from build123d import *

# Parameters (mm, degrees)
ESQUISSE1_W                = 393.7
ESQUISSE1_H                = 95.25
BOSS_EXTRU_1_DEPTH         = 6.35
ESQUISSE2_W                = 38.1
ESQUISSE2_H                = 6.35
ENL_V_MAT_EXTRU_1_DEPTH    = 6.35
ESQUISSE3_W                = 38.1
ESQUISSE3_H                = 6.35
ENL_V_MAT_EXTRU_2_DEPTH    = 6.35
R_P_TITION_LIN_AIRE1_COUNT = 4
R_P_TITION_LIN_AIRE1_PITCH = 76.2
SYM_TRIE2_COPY_1_SKETCH_W  = 38.1
SYM_TRIE2_COPY_1_SKETCH_H  = 6.35
SYM_TRIE2_COPY_1_DEPTH     = 6.35
SYM_TRIE2_COPY_2_SKETCH_W  = 38.1
SYM_TRIE2_COPY_2_SKETCH_H  = 6.35
SYM_TRIE2_COPY_2_DEPTH     = 6.35
SYM_TRIE2_COPY_3_SKETCH_W  = 38.1
SYM_TRIE2_COPY_3_SKETCH_H  = 6.35
SYM_TRIE2_COPY_3_DEPTH     = 6.35


with BuildPart() as part:
    # Esquisse1 → Boss.-Extru.1 (new body)
    with BuildSketch(Plane(origin=(0, 0, 0), x_dir=(1, 0, 0), z_dir=(0, 1, 0))):
        Rectangle(ESQUISSE1_W, ESQUISSE1_H)
    extrude(amount=BOSS_EXTRU_1_DEPTH)

    # Esquisse2 → Enlèv. mat.-Extru.1 (cut)
    with BuildSketch(Plane.ZY.offset(196.85)):
        with Locations((0, 3.175)):
            Rectangle(ESQUISSE2_W, ESQUISSE2_H)
    enl_v_mat_extru_1 = extrude(amount=-ENL_V_MAT_EXTRU_1_DEPTH, mode=Mode.SUBTRACT)

    # Symétrie1: Enlèv. mat.-Extru.1 across plane
    add(enl_v_mat_extru_1.mirror(Plane(origin=(0, 0, 0), x_dir=(0, 0, 1), z_dir=(1, 0, 0))), mode=Mode.SUBTRACT)

    # Esquisse3 → Enlèv. mat.-Extru.2 (cut)
    with BuildSketch(Plane(origin=(0, 0, -47.625), x_dir=(-1, 0, 0), z_dir=(0, 0, -1))):
        with Locations((114.3, 3.175)):
            Rectangle(ESQUISSE3_W, ESQUISSE3_H)
    enl_v_mat_extru_2 = extrude(amount=-ENL_V_MAT_EXTRU_2_DEPTH, mode=Mode.SUBTRACT)

    # Répétition linéaire1: Enlèv. mat.-Extru.2 ×4
    with Locations(*[(i * R_P_TITION_LIN_AIRE1_PITCH, 0, 0) for i in range(1, R_P_TITION_LIN_AIRE1_COUNT)]):
        add(enl_v_mat_extru_2, mode=Mode.SUBTRACT)

    # Symétrie2: Enlèv. mat.-Extru.2 across plane
    add(enl_v_mat_extru_2.mirror(Plane.XY), mode=Mode.SUBTRACT)

    # Symétrie2 copy 1 sketch → Symétrie2 copy 1 (cut)
    with BuildSketch(Plane(origin=(76.2, 0, 47.625), x_dir=(-1, 0, 0), z_dir=(0, 0, 1))):
        with Locations((114.3, -3.175)):
            Rectangle(SYM_TRIE2_COPY_1_SKETCH_W, SYM_TRIE2_COPY_1_SKETCH_H)
    extrude(amount=-SYM_TRIE2_COPY_1_DEPTH, mode=Mode.SUBTRACT)

    # Symétrie2 copy 2 sketch → Symétrie2 copy 2 (cut)
    with BuildSketch(Plane(origin=(152.4, 0, 47.625), x_dir=(-1, 0, 0), z_dir=(0, 0, 1))):
        with Locations((114.3, -3.175)):
            Rectangle(SYM_TRIE2_COPY_2_SKETCH_W, SYM_TRIE2_COPY_2_SKETCH_H)
    extrude(amount=-SYM_TRIE2_COPY_2_DEPTH, mode=Mode.SUBTRACT)

    # Symétrie2 copy 3 sketch → Symétrie2 copy 3 (cut)
    with BuildSketch(Plane(origin=(228.6, 0, 47.625), x_dir=(-1, 0, 0), z_dir=(0, 0, 1))):
        with Locations((114.3, -3.175)):
            Rectangle(SYM_TRIE2_COPY_3_SKETCH_W, SYM_TRIE2_COPY_3_SKETCH_H)
    extrude(amount=-SYM_TRIE2_COPY_3_DEPTH, mode=Mode.SUBTRACT)


solid = part.part
Geometry check sheet. Reference: the model listing, model coordinates, mm. A direction names the side the tool comes from. Coordinates: 2 decimals unless noted, no trailing zeros. Order: outer loops, then holes, each group sorted by start corner. A loop starts at its lowest first (then second) coordinate and runs counter-clockwise, first axis right, second up. Notation, with made-up numbers: (40.25, -13) - (48.25, -13) arc R18 ccw to (48.25, -1) - close; hole circle Ø3 at (46, -16.75). An arc over 180 degrees is marked (long way). One line per item, written item: value.
(1) Sectioned sample at B-B (z = 1). Enter the section's corners in (x, y).
Data:
outline: (-190.5, 0) - (190.5, 0) - (190.5, 6.35) - (-190.5, 6.35) - close
(2) Release check for a two-part mould opening along Z. For faces 1 (the face through (194, 3, 19.05)), 2 (the face through (194, 3, -19.05)), 3 (the face through (-114, 3, 41.275)), 4 (the face through (-95.25, 3, -44)) record: +Z half, -Z half, draft (parallel to the pull), parting line (faces both ways), or undercut.
Data:
face 1: undercut
face 2: undercut
face 3: +Z half
face 4: draft
(3) Thickness scan on probe 1 along X at (y, z) = (3.25, 44.5); probe 2 along X at (y, z) = (4.25, 16.5). Record the ranges inside material, lowest first. Write a range as from..to.
Data:
probe 1: x = -196.85..-133.35, -95.25..-57.15, -19.05..19.05, 57.15..95.25, 133.35..196.85
probe 2: x = -190.5..190.5
(4) Access from +Z, -Z, +X, -X, +Y, -Y to the whole of each face (thin tool, end or side, straight path). Record for faces 5 (the face through (-38, 3, 41.275)), 6 (the face through (0, 3, 47.625)), 7 (the face through (115, 3, -41.275)).
Data:
face 5: +Z, +Y, -Y
face 6: +Z, +X, -X, +Y, -Y
face 7: -Z, +Y, -Y
(5) Sectioned sample at A-A (x = 107). Enter the section's corners in (y, z) (3 decimals).
Data:
outline: (0, -41.275) - (6.35, -41.275) - (6.35, 41.275) - (0, 41.275) - close
(6) Depth check by flat-ended pin: pin 1 Ø3 at (y, z) = (2.5, -1.5) entering from +X; pin 2 Ø1.9 at (x, y) = (-109.5, 2) entering from +Z (3 decimals); pin 3 Ø1.5 at (y, z) = (2.5, -14) entering from -X. Enter the tip coordinate at first touch or a pass-through.
Data:
pin 1: stops at x = 190.5
pin 2: stops at z = 41.275
pin 3: stops at x = -190.5
